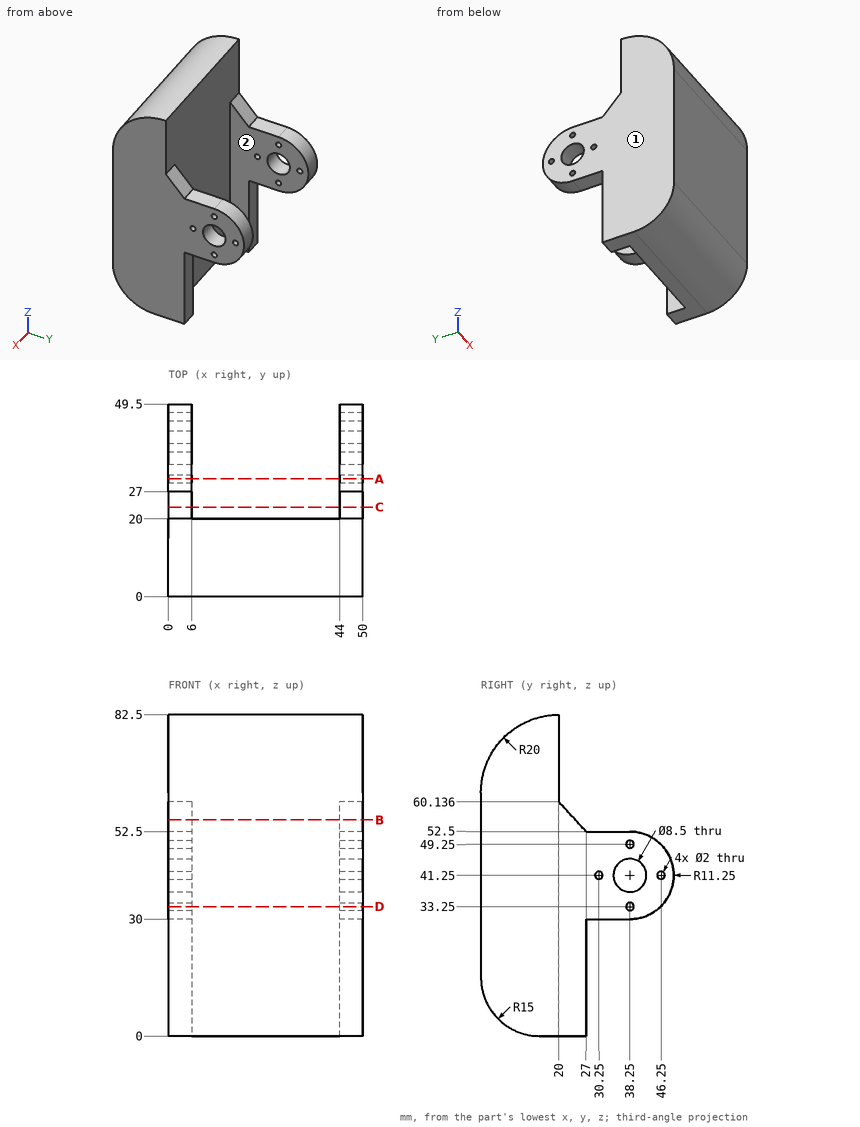
Source: three-view drawing plus pictorial views. Frame: mm from the lowest corner of the part. A direction names the side the tool comes from. Give positions to 0.01 mm unless a question says otherwise; leave off trailing zeros. Loops run counter-clockwise (first coordinate to the right, second up) from the corner with the lowest first, then second, coordinate; pieces in that order, holes last. Notation, with made-up numbers: (55.25, 16.25) -> (74.25, 16.25) arc R20 cw to (74.25, 34.25) -> close; hole circle Ø1 at (44, -36). An arc over 180 degrees is marked (long way). Use a Markdown table: item, result. Add a question column.
(1) Section query B-B (z = 55.5). Output: boundary loops of the cut face in (x, y).
(2) Section query A-A (y = 30.25). Output: boundary loops of the cut face in (x, z), then the cut area to 3 significant figures.
(3) Ray query, line 1 (Z direction, x = 2.8, y = 30.25); line 2 (Z direction, x = 1.65, y = 38.25); line 3 (X direction, y = 35, z = 35.5). Return the intervals inside material, ascending.
(4) Section query D-D (z = 33.25). Output: boundary loops of the cut face in (x, y), then the cut area to 3 significant figures.
(5) First-contact query: pin 1 Ø10 at (x, z) = (13, 65) entering from +Y; pin 2 Ø7 at (y, z) = (38.25, 41.25) entering from +X; pin 3 Ø3 at (x, y) = (4, 33) entering from -Z; pin 4 Ø1.8 at (x, y) = (2, 33.5) entering from +Z. Flat tips, straight axial feed; report the tip coordinate or a pass-through.
(6) Section query C-C (y = 23). Output: boundary loops of the cut face in (x, z).
(7) Access query for the marked faces 1 and 2. Directions: +Z, -Z, +X, -X, +Y, -Y. A direction counts if a zero-diameter tool reaches every point of the face in a straight line with its end or side. Return the directions, or none.
Checked values:
| question | item | result |
|---|---|---|
| 1 | outline | (0, 0) -> (50, 0) -> (50, 24.25) -> (44, 24.25) -> (44, 20) -> (6, 20) -> (6, 24.25) -> (0, 24.25) -> close |
| 2 | outline | (0, 30) -> (6, 30) -> (6, 40.25) -> (0, 40.25) -> close; (0, 42.25) -> (6, 42.25) -> (6, 52.5) -> (0, 52.5) -> close; (44, 30) -> (50, 30) -> (50, 40.25) -> (44, 40.25) -> close; (44, 42.25) -> (50, 42.25) -> (50, 52.5) -> (44, 52.5) -> close |
| 2 | area | 246 mm^2 |
| 3 | line 1 | 30 to 40.25, 42.25 to 52.5 |
| 3 | line 2 | 30 to 32.25, 34.25 to 37, 45.5 to 48.25, 50.25 to 52.5 |
| 3 | line 3 | 0 to 6, 44 to 50 |
| 4 | outline | (0, 0) -> (50, 0) -> (50, 37.25) -> (44, 37.25) -> (44, 20) -> (6, 20) -> (6, 37.25) -> (0, 37.25) -> close; (0, 39.25) -> (6, 39.25) -> (6, 46.16) -> (0, 46.16) -> close; (44, 39.25) -> (50, 39.25) -> (50, 46.16) -> (44, 46.16) -> close |
| 4 | area | 1,290 mm^2 |
| 5 | pin 1 | y = 20 |
| 5 | pin 2 | through |
| 5 | pin 3 | z = 30 |
| 5 | pin 4 | z = 52.5 |
| 6 | outline | (0, 0) -> (6, 0) -> (6, 56.86) -> (0, 56.86) -> close; (44, 0) -> (50, 0) -> (50, 56.86) -> (44, 56.86) -> close |
| 7 | face 1 | +Z, -Z, -X, +Y, -Y |
| 7 | face 2 | +Z, -Z, +Y |
